```python
from build123d import *

# Parameters (mm, degrees)
SKETCH_1_R      = 6.525
SKETCH_1_R_2    = 1.6
EXTRUDE_1_DEPTH = 3


with BuildPart() as part:
    # ｽｹｯﾁ1 → ﾎﾞｽ - 押し出し1 (new body)
    with BuildSketch(Plane.XY):
        with BuildLine():
            Line((-8.356610944, 6.357440801), (-33.979338545, -27.322647238))
            ThreePointArc((-33.979338545, -27.322647238), (-34.479774761, -32.570724678), (-30, -35.35))
            Line((-30, -35.35), (30, -35.35))
            ThreePointArc((30, -35.35), (34.479774761, -32.570724678), (33.979338545, -27.322647238))
            Line((33.979338545, -27.322647238), (8.356610944, 6.357440801))
            ThreePointArc((8.356610944, 6.357440801), (0, 10.5), (-8.356610944, 6.357440801))
        make_face()
        Circle(SKETCH_1_R, mode=Mode.SUBTRACT)
        with Locations((-30, -30.35)):
            Circle(SKETCH_1_R_2, mode=Mode.SUBTRACT)
        with Locations(Location((30, -30.35, 0), (0, 0, 180))):
            Circle(SKETCH_1_R_2, mode=Mode.SUBTRACT)
    extrude(amount=EXTRUDE_1_DEPTH)


solid = part.part
```
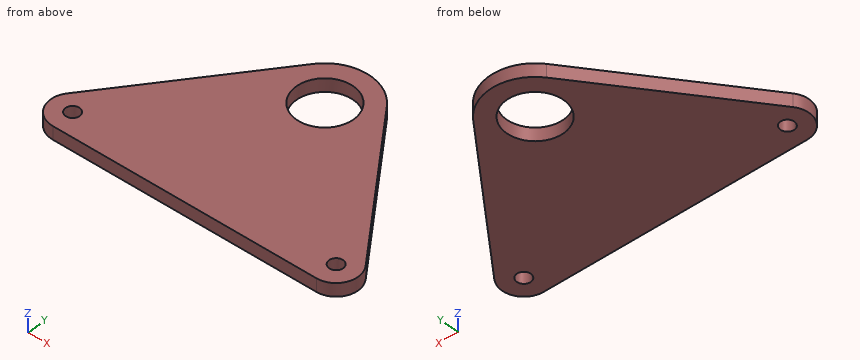
Could you check a few things on this model? Use its own coordinates, in mm. Coordinates: 2 decimals unless noted, no trailing zeros. Write each loop counter-clockwise with the first axis right and the second up, starting at its lowest first coordinate (ties: lowest second). Pieces come first, ordered by that corner, then holes. Notation, with made-up numbers: M -20.75,57 L -13.75,57 A8 ccw -13.75,70 Z; hole C 18.25,83 d5. An arc over 180 degrees is marked long. Answer as CSV lines item,"result". Start each with the question number.
1) I want a section at B-B, the plane y = -30.35. Please give me the cut outline in (x, z), and give its area (3 significant figures).
2) I want a section at C-C, the plane z = 1.8. Please give me the cut outline in (x, y) (3 decimals), and give its area (3 significant figures).
3) Please list where these lines run through material, in increasing order: line 1 (Y direction, x = -30, z = 0.95); line 2 (X direction, y = -5.5, z = 0.25); line 3 (Y direction, x = 29, z = 2.2). Write a range as from..to.
4) I want a section at D-D, the plane x = -18. Please give me the cut outline in (y, z).
5) I want a section at A-A, the plane x = 0. Please give me the cut outline in (y, z) (3 decimals).
Data:
1,outline,"M -35,0 L -31.6,0 L -31.6,3 L -35,3 Z; M -28.4,0 L 28.4,0 L 28.4,3 L -28.4,3 Z; M 31.6,0 L 35,0 L 35,3 L 31.6,3 Z"
1,area,"191 mm^2"
2,outline,"M -33.979,-27.323 A5 ccw -30,-35.35 L 30,-35.35 A5 ccw 33.979,-27.323 L 8.357,6.357 A10.5 ccw -8.357,6.357 Z; hole C -30,-30.35 d3.2; hole C 0,0 d13.05; hole C 30,-30.35 d3.2"
2,area,"1,870 mm^2"
3,line 1,"y = -35.35..-31.95, -28.75..-22.09"
3,line 2,"x = -17.38..-3.51, 3.51..17.38"
3,line 3,"y = -35.35..-31.6, -29.1..-20.78"
4,outline,"M -35.35,0 L -6.32,0 L -6.32,3 L -35.35,3 Z"
5,outline,"M -35.35,0 L -6.525,0 L -6.525,3 L -35.35,3 Z; M 6.525,0 L 10.5,0 L 10.5,3 L 6.525,3 Z"
